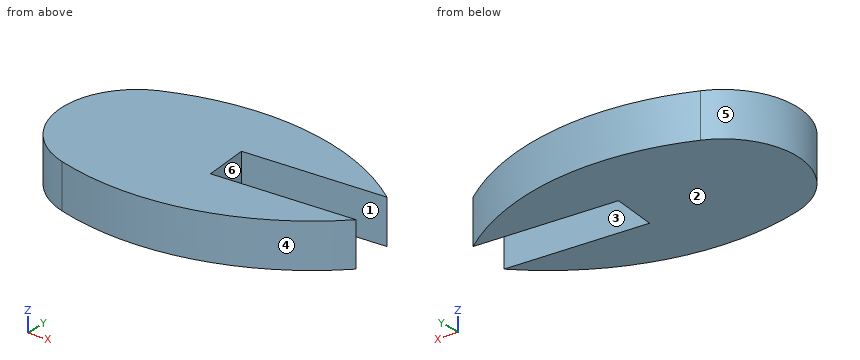
from build123d import *

# Parameters (mm, degrees)
BASE_EXTRUDE_DEPTH = 3


with BuildPart() as part:
    # Sketch1 → Base-Extrude (new body)
    with BuildSketch(Plane.XY):
        with BuildLine():
            Line((-856.474214644, -32.641915538), (-865.720770196, -33.480229749))
            Line((-865.720770196, -33.480229749), (-865.991646191, -30.492483743))
            Line((-865.991646191, -30.492483743), (-856.745090639, -29.654169532))
            ThreePointArc((-856.745090639, -29.654169532), (-864.946405641, -26.511655783), (-873.609416526, -27.957063286))
            ThreePointArc((-873.609416526, -27.957063286), (-876.500341632, -32.951378616), (-872.758344407, -37.344337795))
            ThreePointArc((-872.758344407, -37.344337795), (-863.976635131, -37.208166435), (-856.474214644, -32.641915538))
        make_face()
    extrude(amount=BASE_EXTRUDE_DEPTH)


solid = part.part
The model under review builds one solid part; all positions refer to its coordinate system, in mm. Face numbers are marked on the shaded views. A direction names the side the tool comes from. Give positions to 0.01 mm unless a question says otherwise; leave off trailing zeros. Order: outer loops, then holes, each group sorted by start corner. A loop starts at its lowest first (then second) coordinate and runs counter-clockwise, first axis right, second up. Notation, with made-up numbers: M -1,-36 L 45,-36 A27 ccw 45,-11 Z; hole C 70.25,82 d4. An arc over 180 degrees is marked long. One line per question, with ' | ' between items. Start each with the question number.
1) Consider section C-C, the plane z = 0.55. Give the boundary of the cut face in (x, y), then the cut area to 3 significant figures.
2) Consider section A-A, the plane x = -863. Give the boundary of the cut face in (y, z).
3) Mouldability with a two-part tool opening along X and no side actions: class the marked faces 4, 5 and 6 as pulls with the +X half, pulls with the -X half, needs draft (parallel to the pull), parting line crosses it, or undercut.
4) Consider section D-D, the plane x = -871. Give the boundary of the cut face in (y, z), then the cut area to 3 significant figures.
5) Wall thickness on L1, parallel to Y at x = -861, z = 1.1; L2, parallel to Y at x = -861.25, z = 1.4; L3, parallel to Y at x = -872, z = 1.1: over which ranges is each line inside the solid? List them lowest first. Write a range as from..to.
6) For the marked faces 1, 2 and 3, list the 3-axis set-ups (+Z, -Z, +X, -X, +Y, -Y) from which the entire face can be reached by the end or side of a thin tool; tool diameter is ignored.
7) Consider section B-B, the plane y = -33. Give the boundary of the cut face in (x, z), then the cut area to 3 significant figures.
Found:
1) outline: M -873.61,-27.96 A5 ccw -872.76,-37.34 A16.73 ccw -856.47,-32.64 L -865.72,-33.48 L -865.99,-30.49 L -856.75,-29.65 A16.73 ccw Z | area: 151 mm²
2) outline: M -36.89,0 L -33.23,0 L -33.23,3 L -36.89,3 Z; M -30.22,0 L -26.82,0 L -26.82,3 L -30.22,3 Z
3) face 4: parting line crosses it | face 5: pulls with the -X half | face 6: undercut
4) outline: M -37.69,0 L -27.01,0 L -27.01,3 L -37.69,3 Z | area: 32.1 mm²
5) L1: y = -36.03..-33.05, -30.04..-27.4 | L2: y = -36.15..-33.07, -30.06..-27.31 | L3: y = -37.52..-27.32
6) face 1: +Z, -Z, +X | face 2: -Z, +X, -X, +Y, -Y | face 3: +Z, -Z
7) outline: M -876.5,0 L -865.76,0 L -865.76,3 L -876.5,3 Z; M -860.42,0 L -856.82,0 L -856.82,3 L -860.42,3 Z | area: 43.0 mm²
